Here's how the part is built. I have some questions about the finished solid (model axes, mm). A direction names the side the tool comes from. Coordinates: 2 decimals unless noted, no trailing zeros. Write each loop counter-clockwise with the first axis right and the second up, starting at its lowest first coordinate (ties: lowest second). Pieces come first, ordered by that corner, then holes. Notation, with made-up numbers: M 31.5,39.25 L 63.5,39.25 A36 cw 63.5,77.25 Z; hole C 86.5,10.5 d7. An arc over 180 degrees is marked long. Use a Markdown table: item, result.
```python
from build123d import *

# Parameters (mm, degrees)
CROQUIS1_R              = 14
CROQUIS1_R_2            = 4
SALIENTE_EXTRUIR1_DEPTH = 5
CROQUIS2_R              = 12
CROQUIS2_R_2            = 11
SALIENTE_EXTRUIR2_DEPTH = 3.5


with BuildPart() as part:
    # Croquis1 → Saliente-Extruir1 (new body)
    with BuildSketch(Plane(origin=(0, 0, 0), x_dir=(0, 0, -1), z_dir=(1, 0, 0))):
        Circle(CROQUIS1_R)
        Circle(CROQUIS1_R_2, mode=Mode.SUBTRACT)
    extrude(amount=SALIENTE_EXTRUIR1_DEPTH)

    # Croquis2 → Saliente-Extruir2 (add)
    with BuildSketch(Plane.ZY):
        Circle(CROQUIS2_R)
        Circle(CROQUIS2_R_2, mode=Mode.SUBTRACT)
    extrude(amount=SALIENTE_EXTRUIR2_DEPTH)


solid = part.part
```
1. I need wall thicknesses on probe 1 along Y at (x, z) = (3.2, 0); probe 2 along X at (y, z) = (4.5, -3.75); probe 3 along Y at (x, z) = (-2.3, 0). Which ranges of each line are inside material? Lowest first, please.
Answers follow:
| item | result |
|---|---|
| probe 1 | y = -14 to -4, 4 to 14 |
| probe 2 | x = 0 to 5 |
| probe 3 | y = -12 to -11, 11 to 12 |
2. Suppose I cut it at A-A on z = 0. Write out the boundary of the cut face in (x, y), and give its area (3 significant figures).
Answers follow:
| item | result |
|---|---|
| outline | M -3.5,-12 L 0,-12 L 0,-14 L 5,-14 L 5,-4 L 0,-4 L 0,-11 L -3.5,-11 Z; M -3.5,11 L 0,11 L 0,4 L 5,4 L 5,14 L 0,14 L 0,12 L -3.5,12 Z |
| area | 107 mm2 |
3. We'd pull the mould along Z, two halves only. Please class faces 1 (the face through (0, -5, 0)), 2 (the face through (-1.73, 0.53, -11.99)), 3 (the face through (5, -3, -3)): +Z half, -Z half, draft (parallel to the pull), parting line (faces both ways), or undercut.
Answers follow:
| item | result |
|---|---|
| face 1 | undercut |
| face 2 | parting line |
| face 3 | draft |
4. Suppose I cut it at D-D on y = -7.75. Write out the boundary of the cut face in (x, z), and give its area (3 significant figures).
Answers follow:
| item | result |
|---|---|
| outline | M -3.5,-9.16 L 0,-9.16 L 0,-11.66 L 5,-11.66 L 5,11.66 L 0,11.66 L 0,9.16 L -3.5,9.16 L -3.5,7.81 L 0,7.81 L 0,-7.81 L -3.5,-7.81 Z |
| area | 126 mm2 |
5. Will these pins go through, and if not, where does the flat tip stop? pin 1 Ø1.5 at (x, y) = (-2, -4.5) entering from +Z; pin 2 Ø11 at (y, z) = (3, -2) entering from -X; pin 3 Ø4 at (x, y) = (3, -9) entering from +Z.
Answers follow:
| item | result |
|---|---|
| pin 1 | stops at z = 11.4 |
| pin 2 | stops at x = 0 |
| pin 3 | stops at z = 12.12 |
6. Which directions (+Z, -Z, +X, -X, +Y, -Y) give clear straight access to the entire face, cutting with the end or side of a thin tool? Please do faces 4 (the face through (-3.5, -10, 5)), 5 (the face through (0, 10.4, 6.3)).
Answers follow:
| item | result |
|---|---|
| face 4 | +Z, -Z, -X, +Y, -Y |
| face 5 | -X |
7. Suppose I cut it at C-C on x = 4. Write out the boundary of the cut face in (y, z), and give its area (3 significant figures).
Answers follow:
| item | result |
|---|---|
| outline | C 0,0 d28; hole C 0,0 d8 |
| area | 565 mm2 |
